Source: CAD feature listing. Evaluate the final solid. Frame: model axes, mm. Face numbers are marked on the shaded views. A direction names the side the tool comes from. Give positions to 0.01 mm unless a question says otherwise; leave off trailing zeros. Order: outer loops, then holes, each group sorted by start corner. A loop starts at its lowest first (then second) coordinate and runs counter-clockwise, first axis right, second up. Notation, with made-up numbers: M 51.25,-21 L 103.25,-21 A28 ccw 103.25,9 Z; hole C 49,-15.5 d9. An arc over 180 degrees is marked long. Answer in a Markdown table with one row per item. Add a question column.
(1) Pin query (flat end, axial travel): P1, Ø5.5, axis at x = 11, y = -17.5, coming from the -Z side; P2, Ø3, axis at x = 14.5, z = 3, coming from the +Y side; P3, Ø4, axis at x = 32.5, z = 4, coming from the -Y side; P4, Ø4, axis at y = -11.5, z = 10, coming from the -X side. Return the tip coordinate at first contact, or that it passes through.
(2) Material intervals for line 1 along X through (y, z) = (11, 5.25); line 2 along Y through (x, z) = (39.5, 8.5); line 3 along Y through (x, z) = (11, 2.5), sorted ascending.
(3) Section query B-B, the plane x = 39.5. Return loops of the section in (y, z).
(4) Set-up query: the marked faces 1, 2, 3 and 4. Return all of +Z, -Z, +X, -X, +Y, -Y with unobstructed straight access to the full face (end or side cutting, diameter ignored); none if empty.
(5) Section query C-C, the plane y = -5. Return loops of the section in (x, z).
(6) Section query A-A, the plane z = 4. Return loops of the section in (x, y), plus the area to 3 significant figures.
from build123d import *

# Parameters (mm, degrees)
RECTANGLE003_W       = 22
RECTANGLE003_H       = 13
PAD_DEPTH            = 12
RECTANGLE002_FACE1_W = 22
RECTANGLE002_FACE1_H = 24
PAD002_DEPTH         = 4
RECTANGLE_FACE1_W    = 46
RECTANGLE_FACE1_H    = 22
PAD003_DEPTH         = 4
RECTANGLE001_W       = 13
RECTANGLE001_H       = 22
PAD004_DEPTH         = 12
CIRCLE002_R          = 2.2
POCKET_DEPTH         = 22
CIRCLE_EDGE1_R       = 3
POCKET001_DEPTH      = 5
CIRCLE001_R          = 2.2
POCKET002_DEPTH      = 22
POCKET003_DEPTH      = 22
POCKET004_DEPTH      = 22
CHAMFER_SIZE         = 2
CHAMFER001_SIZE      = 1.7
CHAMFER002_SIZE      = 1.7
FILLET_R             = 1.5


with BuildPart() as part:
    # Rectangle003 → Pad (new body)
    with BuildSketch(Plane(origin=(0, -24, 0), x_dir=(1, 0, 0), z_dir=(0, 0, 1))):
        with Locations((11, 6.5)):
            Rectangle(RECTANGLE003_W, RECTANGLE003_H)
    extrude(amount=PAD_DEPTH)

    # Rectangle002 Face1 → Pad002 (add)
    with BuildSketch(Plane(origin=(0, -24, 0), x_dir=(1, 0, 0), z_dir=(0, 0, 1))):
        with Locations((11, 12)):
            Rectangle(RECTANGLE002_FACE1_W, RECTANGLE002_FACE1_H)
    extrude(amount=-PAD002_DEPTH)

    # Rectangle Face1 → Pad003 (add)
    with BuildSketch(Plane.XY):
        with Locations((23, 11)):
            Rectangle(RECTANGLE_FACE1_W, RECTANGLE_FACE1_H)
    extrude(amount=-PAD003_DEPTH)

    # Rectangle001 → Pad004 (join)
    with BuildSketch(Plane(origin=(33, 0, 0), x_dir=(1, 0, 0), z_dir=(0, 0, 1))):
        with Locations((6.5, 11)):
            Rectangle(RECTANGLE001_W, RECTANGLE001_H)
    extrude(amount=PAD004_DEPTH)

    # Circle002 → Pocket (cut)
    with BuildSketch(Plane(origin=(11, -17.5, 0), x_dir=(1, 0, 0), z_dir=(0, 0, 1))):
        Circle(CIRCLE002_R)
    extrude(amount=-POCKET_DEPTH, mode=Mode.SUBTRACT)

    # Circle Edge1 → Pocket001 (cut)
    with BuildSketch(Plane(origin=(8, 14, 0), x_dir=(1, 0, 0), z_dir=(0, 0, 1))):
        Circle(CIRCLE_EDGE1_R)
    extrude(amount=-POCKET001_DEPTH, mode=Mode.SUBTRACT)

    # Circle001 → Pocket002 (cut)
    with BuildSketch(Plane(origin=(39.5, 11, 0), x_dir=(1, 0, 0), z_dir=(0, 0, 1))):
        Circle(CIRCLE001_R)
    extrude(amount=-POCKET002_DEPTH, mode=Mode.SUBTRACT)

    # Circle001 → Pocket003 (cut)
    with BuildSketch(Plane(origin=(39.5, 11, 0), x_dir=(1, 0, 0), z_dir=(0, 0, 1))):
        Circle(CIRCLE001_R)
    extrude(amount=POCKET003_DEPTH, mode=Mode.SUBTRACT)

    # Circle002 → Pocket004 (cut)
    with BuildSketch(Plane(origin=(11, -17.5, 0), x_dir=(1, 0, 0), z_dir=(0, 0, 1))):
        Circle(CIRCLE002_R)
    extrude(amount=POCKET004_DEPTH, mode=Mode.SUBTRACT)

    # Chamfer
    chamfer_edges = [part.edges().sort_by_distance(p)[0] for p in [
        (5, 14, -4),
    ]]
    chamfer(chamfer_edges, length=CHAMFER_SIZE)

    # Chamfer001
    chamfer001_edges = [part.edges().sort_by_distance(p)[0] for p in [
        (37.3, 11, -4),
    ]]
    chamfer(chamfer001_edges, length=CHAMFER001_SIZE)

    # Chamfer002
    chamfer002_edges = [part.edges().sort_by_distance(p)[0] for p in [
        (8.8, -17.5, -4),
    ]]
    chamfer(chamfer002_edges, length=CHAMFER002_SIZE)

    # Fillet
    fillet_edges = [part.edges().sort_by_distance(p)[0] for p in [
        (0, -24, 4),
        (0, -17.5, 12),
        (0, -11, 6),
        (0, -1, -4),
        (11, -24, -4),
        (22, -24, 4),
        (11, -24, 12),
        (11, -11, 12),
        (22, -17.5, 12),
        (33, 0, 6),
        (39.5, 0, 12),
        (46, 0, 4),
        (46, 11, 12),
        (33, 11, 12),
        (39.5, 22, 12),
        (33, 22, 6),
        (0, 22, -2),
        (22, -11, 6),
        (46, 22, 4),
        (46, 11, -4),
        (23, 22, -4),
        (34, 0, -4),
        (22, -12, -4),
    ]]
    fillet(fillet_edges, radius=FILLET_R)


solid = part.part
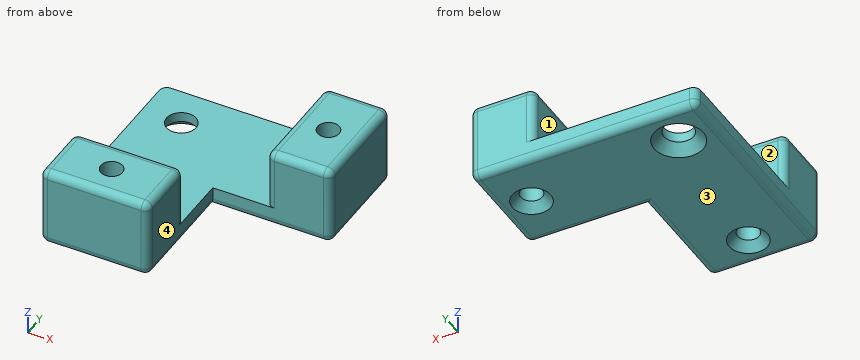
Values follow:
| question | item | result |
|---|---|---|
| 1 | P1 | stops at z = -2.85 |
| 1 | P2 | stops at y = -11 |
| 1 | P3 | stops at y = 0 |
| 1 | P4 | stops at x = 0 |
| 2 | line 1 | x = 33 to 37.3, 41.7 to 46 |
| 2 | line 2 | y = 0 to 8.8, 13.2 to 22 |
| 2 | line 3 | y = -24 to -19.7, -15.3 to -11 |
| 3 | outline | M 0,-2.5 A1.5 ccw 1.5,-4 L 7.1,-4 L 8.8,-2.3 L 8.8,12 L 1.5,12 A1.5 ccw 0,10.5 Z; M 13.2,-2.3 L 14.9,-4 L 20.5,-4 A1.5 ccw 22,-2.5 L 22,10.5 A1.5 ccw 20.5,12 L 13.2,12 Z |
| 4 | face 1 | +Z, -X, +Y, -Y |
| 4 | face 2 | +Z, +X, -X, +Y |
| 4 | face 3 | -Z, +X, -X, +Y, -Y |
| 4 | face 4 | +Z, -Z, +X, -Y |
| 5 | outline | M 0,-2.5 A1.5 ccw 1.5,-4 L 20.5,-4 A1.5 ccw 22,-2.5 L 22,0 L 0,0 Z |
| 6 | outline | M 0,-22.5 A1.5 ccw 1.5,-24 L 20.5,-24 A1.5 ccw 22,-22.5 L 22,-12.5 A1.5 ccw 20.5,-11 L 1.5,-11 A1.5 ccw 0,-12.5 Z; M 33,1.5 A1.5 ccw 34.5,0 L 44.5,0 A1.5 ccw 46,1.5 L 46,20.5 A1.5 ccw 44.5,22 L 34.5,22 A1.5 ccw 33,20.5 Z; hole C 11,-17.5 d4.4; hole C 39.5,11 d4.4 |
| 6 | area | 538 mm² |
